The model under review builds one solid part; all positions refer to its coordinate system, in mm. Round coordinates to 2 decimals unless told otherwise and drop trailing zeros. Write each loop counter-clockwise with the first axis right and the second up, starting at its lowest first coordinate (ties: lowest second). Pieces come first, ordered by that corner, then holes. Notation, with made-up numbers: M -9,58.5 L 0,58.5 A15 ccw 0,79.5 Z; hole C 89.5,30 d2. An arc over 180 degrees is marked long. One line per item, written item: value. Start each with the question number.
1) Take a section at B-B, the plane x = -86. Write out the cut boundary in (y, z), and give its area (3 significant figures).
2) Take a section at D-D, the plane z = 60. Write out the cut boundary in (x, y), and give its area (3 significant figures).
3) Wall thickness on probe 1 along X at (y, z) = (2.55, -53); probe 2 along Z at (x, y) = (86, 1.35); probe 3 along Z at (x, y) = (12.5, 1.6): over which ranges is each line inside the solid? List them lowest first.
4) For P1, Ø2, axis at y = 2.5, z = -14, coming from the +X side; P2, Ø0.9, axis at x = -0.5, y = 1.5, coming from the -Z side; P3, Ø1.5, axis at y = 2, z = 59.5, coming from the +X side, all flat-tipped, find the tip position at first contact; note any pin that passes through.
5) Take a section at A-A, the plane x = 17. Write out the cut boundary in (y, z), and give its area (3 significant figures).
6) Take a section at C-C, the plane y = 3.1. State how many separate pieces and enclosed holes the cut face has, and give its area (3 significant figures).
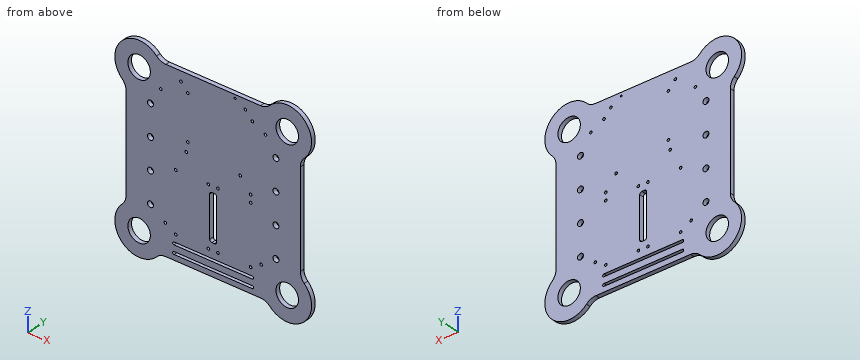
from build123d import *

# Parameters (mm, degrees)
SKETCH1_R          = 12.9
BASE_DEPTH         = 5
SKETCH2_R          = 1.5
SKETCH2_R_2        = 3.4
SKETCH2_R_3        = 1
CUT_EXTRUDE1_DEPTH = 6
CUT_EXTRUDE2_DEPTH = 6
SKETCH4_R          = 1.5
CUT_EXTRUDE3_DEPTH = 6


with BuildPart() as part:
    # Sketch1 → Base (new body)
    with BuildSketch(Plane(origin=(0, 0, 0), x_dir=(1, 0, 0), z_dir=(0, 1, 0))):
        with BuildLine():
            Line((0, 100), (54.333894933, 100))
            ThreePointArc((54.333894933, 100), (60.150136961, 101.173527975), (65.056309292, 104.51048951))
            ThreePointArc((65.056309292, 104.51048951), (104.728279195, 104.728279195), (104.51048951, 65.056309292))
            ThreePointArc((104.51048951, 65.056309292), (101.173527975, 60.150136961), (100, 54.333894933))
            Line((100, 54.333894933), (100, -54.333894933))
            ThreePointArc((100, -54.333894933), (101.173527975, -60.150136961), (104.51048951, -65.056309292))
            ThreePointArc((104.51048951, -65.056309292), (104.728279195, -104.728279195), (65.056309292, -104.51048951))
            ThreePointArc((65.056309292, -104.51048951), (60.150136961, -101.173527975), (54.333894933, -100))
            Line((54.333894933, -100), (0, -100))
            Line((0, -100), (0, 81))
            Line((0, 81), (45, 81))
            ThreePointArc((45, 81), (46.5, 82.5), (45, 84))
            Line((45, 84), (0, 84))
            Line((0, 84), (0, 91))
            Line((0, 91), (45, 91))
            ThreePointArc((45, 91), (46.5, 92.5), (45, 94))
            Line((45, 94), (0, 94))
            Line((0, 94), (0, 100))
        make_face()
        with Locations((85, 85)):
            Circle(SKETCH1_R, mode=Mode.SUBTRACT)
        with Locations((85, -85)):
            Circle(SKETCH1_R, mode=Mode.SUBTRACT)
    base = extrude(amount=BASE_DEPTH)

    # Mirror1: Base across plane
    add(base.mirror(Plane(origin=(0, 0, 0), x_dir=(0, 0, 1), z_dir=(1, 0, 0))))

    # Sketch2 → Cut-Extrude1 (cut, through all)
    with BuildSketch(Plane(origin=(0, 5, 0), x_dir=(1, 0, 0), z_dir=(0, 1, 0))):
        with Locations((-42.960009902, 72.46)):
            Circle(SKETCH2_R)
        with Locations((-5.460009902, 72.46)):
            Circle(SKETCH2_R)
        with Locations((5.460009902, 72.46)):
            Circle(SKETCH2_R)
        with Locations((42.960009902, 72.46)):
            Circle(SKETCH2_R)
        with Locations((72.009618943, 52.5)):
            Circle(SKETCH2_R_2)
        with Locations((-28.986150524, -79.986157497)):
            Circle(SKETCH2_R)
        with Locations((72.009618943, -17.5)):
            Circle(SKETCH2_R_2)
        with Locations((72.009618943, -52.5)):
            Circle(SKETCH2_R_2)
        with Locations((42.960009902, 5.46)):
            Circle(SKETCH2_R)
        with Locations((42.960009902, -2.986157497)):
            Circle(SKETCH2_R)
        with Locations((5.460009902, 5.46)):
            Circle(SKETCH2_R)
        with Locations((-5.460009902, 5.46)):
            Circle(SKETCH2_R)
        with Locations((-28.986150524, -28.986157497)):
            Circle(SKETCH2_R)
        with Locations((-42.960009902, 5.46)):
            Circle(SKETCH2_R)
        with Locations((-72.009618943, 52.5)):
            Circle(SKETCH2_R_2)
        with Locations((-72.009618943, -17.5)):
            Circle(SKETCH2_R_2)
        with Locations((-72.009618943, -52.5)):
            Circle(SKETCH2_R_2)
        with Locations((45.013849476, -79.986157497)):
            Circle(SKETCH2_R)
        with Locations((36.999763655, -89)):
            Circle(SKETCH2_R)
        with Locations((-37.000236345, -89)):
            Circle(SKETCH2_R)
        with Locations((-72.009618943, 17.5)):
            Circle(SKETCH2_R_2)
        with Locations((72.009618943, 17.5)):
            Circle(SKETCH2_R_2)
        with Locations((25.1, -96)):
            Circle(SKETCH2_R_3)
    extrude(amount=-CUT_EXTRUDE1_DEPTH, mode=Mode.SUBTRACT)

    # Sketch3 → Cut-Extrude2 (cut, through all)
    with BuildSketch(Plane(origin=(0, 5, 0), x_dir=(1, 0, 0), z_dir=(0, 1, 0))):
        with BuildLine():
            Line((0, 64.46), (1.5, 64.46))
            ThreePointArc((1.5, 64.46), (3.267766953, 63.727766953), (4, 61.96))
            Line((4, 61.96), (4, 14.96))
            ThreePointArc((4, 14.96), (3.267766953, 13.192233047), (1.5, 12.46))
            Line((1.5, 12.46), (-1.5, 12.46))
            ThreePointArc((-1.5, 12.46), (-3.267766953, 13.192233047), (-4, 14.96))
            Line((-4, 14.96), (-4, 61.96))
            ThreePointArc((-4, 61.96), (-3.267766953, 63.727766953), (-1.5, 64.46))
            Line((-1.5, 64.46), (0, 64.46))
        make_face()
    extrude(amount=-CUT_EXTRUDE2_DEPTH, mode=Mode.SUBTRACT)

    # Sketch4 → Cut-Extrude3 (cut, through all)
    with BuildSketch(Plane(origin=(0, 5, 0), x_dir=(1, 0, 0), z_dir=(0, 1, 0))):
        with Locations((-55.009618943, 65)):
            Circle(SKETCH4_R)
        with Locations((55.009618943, 65)):
            Circle(SKETCH4_R)
        with Locations((-60.009618943, -72)):
            Circle(SKETCH4_R)
        with Locations((60.009618943, -72)):
            Circle(SKETCH4_R)
        with Locations((31.009618943, -18)):
            Circle(SKETCH4_R)
        with Locations((-31.009618943, -18)):
            Circle(SKETCH4_R)
    extrude(amount=-CUT_EXTRUDE3_DEPTH, mode=Mode.SUBTRACT)


solid = part.part
Checked values:
1. outline: M 0,-112.88 L 5,-112.88 L 5,-97.86 L 0,-97.86 Z; M 0,-72.14 L 5,-72.14 L 5,72.14 L 0,72.14 Z; M 0,97.86 L 5,97.86 L 5,112.88 L 0,112.88 Z
1. area: 872 mm2
2. outline: M -101.11,0 L 101.11,0 L 101.11,5 L -101.11,5 Z
2. area: 1,010 mm2
3. probe 1: x = -100 to -75.37, -68.65 to -4, 4 to 68.65, 75.37 to 100
3. probe 2: z = -112.88 to -97.86, -72.14 to 72.14, 97.86 to 112.88
3. probe 3: z = -100 to -94, -91 to -84, -81 to 100
4. P1: stops at x = 100
4. P2: stops at z = -100
4. P3: stops at x = 101.22
5. outline: M 0,-100 L 5,-100 L 5,-94 L 0,-94 Z; M 0,-91 L 5,-91 L 5,-84 L 0,-84 Z; M 0,-81 L 5,-81 L 5,100 L 0,100 Z
5. area: 970 mm2
6. separate pieces: 1
6. enclosed holes: 36
6. area: 39,800 mm2
